from build123d import *

# Parameters (mm, degrees)
EXTRUDE_1_DEPTH         = 3
SKETCH_3_R              = 7.6
SKETCH_3_R_2            = 9.5
SKETCH_3_R_3            = 1.55
CUT_EXTRUDE_1_DEPTH     = 112.843640856
SKETCH_4_R              = 13.75
CUT_EXTRUDE_2_DEPTH     = 2
EXTRUDE_6_DEPTH         = 3
SKETCH_10_R             = 1.55
CUT_EXTRUDE_3_DEPTH     = 124.991771172
CUT_EXTRUDE_6_DEPTH     = 124.991771172
EXTRUDE_7_DEPTH         = 3
CUT_EXTRUDE_7_DEPTH     = 124.991771172
SKETCH_18_W             = 9.7
SKETCH_18_H             = 35
CUT_EXTRUDE_9_DEPTH     = 124.991771172
SKETCH_19_R             = 1.55
CUT_EXTRUDE_10_DEPTH    = 124.991771172
SKETCH_20_W             = 61.573881036
SKETCH_20_H             = 3.2
SKETCH_20_W_2           = 79.598608315
SKETCH_20_H_2           = 1.2
EXTRUDE_8_DEPTH         = 3
EXTRUDE_START           = -3
EXTRUDE_9_DEPTH         = 3
EXTRUDE_11_DEPTH        = 3
SKETCH_25_R             = 9.5
EXTRUDE_12_DEPTH        = 3
SKETCH_26_R             = 9.5
CUT_EXTRUDE_11_DEPTH    = 124.991771172
EXTRUDE_13_DEPTH        = 3
CUT_EXTRUDE_12_DEPTH    = 3
SKETCH_29_W             = 5.5
SKETCH_29_H             = 32
EXTRUDE_14_DEPTH        = 3
SKETCH_32_W             = 9.716106013
SKETCH_32_H             = 6
CUT_EXTRUDE_13_DEPTH    = 124.991771172
CUT_EXTRUDE_16_DEPTH    = 3
SKETCH_35_W             = 2.5
SKETCH_35_H             = 44.4
EXTRUDE_15_DEPTH        = 3
SKETCH_36_R             = 1.55
CUT_EXTRUDE_14691_DEPTH = 3
EXTRUDE_16_DEPTH        = 3
SKETCH_38_R             = 2.75
CUT_EXTRUDE_L_DEPTH     = 121.232106085
SKETCH_57_R             = 1.55
EXTRUDE_17_DEPTH        = 3
CUT_EXTRUDE_17_DEPTH    = 121.232106085


# Read off the part's stored shape, not the designer's step: 高级异型孔6
with BuildPart() as part:
    # 草图1 → 凸台-拉伸1 (new body)
    with BuildSketch(Plane(origin=(0, 0, 0), x_dir=(0, 0, -1), z_dir=(1, 0, 0))):
        Polygon((0, -50), (18.610302832, -39.45792997), (18.610302832, 40), (58.496702951, 40), (58.496702951, 0), (100, 0), (100, -50), align=None)
    extrude(amount=EXTRUDE_1_DEPTH)

    # 草图3 → 切除-拉伸1 (cut, through all)
    with BuildSketch(Plane.ZY):
        with Locations((-74, -24.961577338)):
            Circle(SKETCH_3_R)
        with Locations((-34.176393222, 0)):
            Circle(SKETCH_3_R_2)
        with Locations((-74, -7.461577338)):
            Circle(SKETCH_3_R_3)
        with Locations((-56.5, -24.961577338)):
            Circle(SKETCH_3_R_3)
        with Locations((-74, -42.461577338)):
            Circle(SKETCH_3_R_3)
        with Locations((-91.5, -24.961577338)):
            Circle(SKETCH_3_R_3)
    extrude(amount=-CUT_EXTRUDE_1_DEPTH, mode=Mode.SUBTRACT)

    # 草图4 → 切除-拉伸2 (cut)
    with BuildSketch(Plane.ZY):
        with Locations((-74, -24.961577338)):
            Circle(SKETCH_4_R)
    extrude(amount=-CUT_EXTRUDE_2_DEPTH, mode=Mode.SUBTRACT)

    # 草图6 → 凸台-拉伸6 (add)
    with BuildSketch(Plane.ZY):
        with BuildLine():
            Line((-102.983893987, -45.2), (-110.983893987, -45.2))
            Line((-110.983893987, -45.2), (-111, -50))
            Line((-111, -50), (-100, -50))
            Line((-100, -50), (-100, 0))
            Line((-100, 0), (-110.983893987, 0))
            Line((-110.983893987, 0), (-110.983893987, -6.8))
            Line((-110.983893987, -6.8), (-102.983893987, -6.8))
            ThreePointArc((-102.983893987, -6.8), (-101.283893987, -8.5), (-102.983893987, -10.2))
            Line((-102.983893987, -10.2), (-110.983893987, -10.2))
            Line((-110.983893987, -10.2), (-110.983893987, -41.8))
            Line((-110.983893987, -41.8), (-102.983893987, -41.8))
            ThreePointArc((-102.983893987, -41.8), (-101.283893987, -43.5), (-102.983893987, -45.2))
        make_face()
        with BuildLine():
            Line((-15.00347976, -50), (-34.686448159, -50))
            ThreePointArc((-34.686448159, -50), (-33.16855591, -50.235967767), (-31.793933119, -50.921598751))
            Line((-31.793933119, -50.921598751), (-26.580472983, -54.619128968))
            ThreePointArc((-26.580472983, -54.619128968), (-25.755699309, -55.030507559), (-24.844963959, -55.172088219))
            ThreePointArc((-24.844963959, -55.172088219), (-23.93422861, -55.030507559), (-23.109454935, -54.619128968))
            Line((-23.109454935, -54.619128968), (-17.8959948, -50.921598751))
            ThreePointArc((-17.8959948, -50.921598751), (-16.521372009, -50.235967767), (-15.00347976, -50))
        make_face()
    extrude(amount=-EXTRUDE_6_DEPTH)

    # 草图10 → 切除-拉伸3 (cut, through all)
    with BuildSketch(Plane.ZY):
        with Locations((-105.983893987, -15.2)):
            Circle(SKETCH_10_R)
        with Locations((-105.983893987, -36.8)):
            Circle(SKETCH_10_R)
    extrude(amount=-CUT_EXTRUDE_3_DEPTH, mode=Mode.SUBTRACT)

    # 草图14 → 切除-拉伸6 (cut, through all)
    with BuildSketch(Plane(origin=(3, 0, 0), x_dir=(0, 0, -1), z_dir=(1, 0, 0))):
        with BuildLine():
            Line((58.496702951, 0), (58.496702951, 40))
            Line((58.496702951, 40), (18.610302832, 40))
            Line((18.610302832, 40), (18.610302832, 18.686206016))
            ThreePointArc((18.610302832, 18.686206016), (44.493983197, 22.023278649), (58.496702951, 0))
        make_face()
    extrude(amount=-CUT_EXTRUDE_6_DEPTH, mode=Mode.SUBTRACT)

    # 草图15 → 凸台-拉伸7 (add)
    with BuildSketch(Plane(origin=(3, 0, 0), x_dir=(0, 0, -1), z_dir=(1, 0, 0))):
        with BuildLine():
            Line((18.610302832, 18.686206016), (18.610302832, -18.686206016))
            ThreePointArc((18.610302832, -18.686206016), (9.856083494, 0), (18.610302832, 18.686206016))
        make_face()
    extrude(amount=-EXTRUDE_7_DEPTH)

    # 草图16 → 切除-拉伸7 (cut, through all)
    with BuildSketch(Plane(origin=(3, 0, 0), x_dir=(0, 0, -1), z_dir=(1, 0, 0))):
        with BuildLine():
            Line((18.610302832, -18.686206016), (18.610302832, 0))
            ThreePointArc((18.610302832, 0), (34.176393222, 15.56609039), (49.742483613, 0))
            Line((49.742483613, 0), (58.496702951, 0))
            ThreePointArc((58.496702951, 0), (23.858803248, 22.023278649), (18.610302832, -18.686206016))
        make_face()
    extrude(amount=-CUT_EXTRUDE_7_DEPTH, mode=Mode.SUBTRACT)

    # 草图18 → 切除-拉伸9 (cut, through all)
    with BuildSketch(Plane.ZY):
        with Locations((-106.133893987, -26)):
            Rectangle(SKETCH_18_W, SKETCH_18_H)
    extrude(amount=-CUT_EXTRUDE_9_DEPTH, mode=Mode.SUBTRACT)

    # 草图19 → 切除-拉伸10 (cut, through all)
    with BuildSketch(Plane.ZY):
        with Locations((-105.983893987, -1.8)):
            Circle(SKETCH_19_R)
        with Locations((-105.993932098, -48.2)):
            Circle(SKETCH_19_R)
    extrude(amount=-CUT_EXTRUDE_10_DEPTH, mode=Mode.SUBTRACT)

    # 草图20 → 凸台-拉伸8 (add)
    with BuildSketch(Plane.ZY):
        with Locations((-80.196953469, 1.6)):
            Rectangle(SKETCH_20_W, SKETCH_20_H)
        with Locations((-71.200695842, -50.6)):
            Rectangle(SKETCH_20_W_2, SKETCH_20_H_2)
    extrude(amount=-EXTRUDE_8_DEPTH)

    # 草图22 → 凸台-拉伸9 (add)
    with BuildSketch(Plane.ZY.offset(EXTRUDE_START)):
        with BuildLine():
            Line((-18.610302832, 0), (-18.610302832, 25))
            Line((-18.610302832, 25), (-41.044918155, 13.968769999))
            ThreePointArc((-41.044918155, 13.968769999), (-25.948784515, 13.213993529), (-18.610302832, 0))
        make_face()
    extrude(amount=EXTRUDE_9_DEPTH)

    # 草图24 → 凸台-拉伸11 (add)
    with BuildSketch(Plane.ZY):
        Polygon((-18.610302832, 25), (-70.983893987, 3.2), (-49.410012951, 3.2), align=None)
    extrude(amount=-EXTRUDE_11_DEPTH)

    # 草图25 → 凸台-拉伸12 (add, through all)
    with BuildSketch(Plane(origin=(3, 0, 0), x_dir=(0, 0, -1), z_dir=(1, 0, 0))):
        with Locations((34.176393222, 0)):
            Circle(SKETCH_25_R)
    extrude(amount=-EXTRUDE_12_DEPTH)

    # 草图26 → 切除-拉伸11 (cut, through all)
    with BuildSketch(Plane(origin=(3, 0, 0), x_dir=(0, 0, -1), z_dir=(1, 0, 0))):
        with Locations((29.059828781, -15.2)):
            Circle(SKETCH_26_R)
    extrude(amount=-CUT_EXTRUDE_11_DEPTH, mode=Mode.SUBTRACT)

    # 草图27 → 凸台-拉伸13 (add)
    with BuildSketch(Plane.ZY):
        Polygon((-18.610302832, -10.2), (-13.610302832, -15.2), (-18.610302832, -20.2), align=None)
    extrude(amount=-EXTRUDE_13_DEPTH)

    # 草图28 → 切除-拉伸12 (cut)
    with BuildSketch(Plane.ZY):
        Polygon((-110.983893987, 3.2), (-101.283893987, 3.2), (-70.983893987, 3.2), (-95.008477086, -6.8), (-101.283893987, -6.8), (-101.283893987, -45.2), (-110.983893987, -45.2), align=None)
    extrude(amount=-CUT_EXTRUDE_12_DEPTH, mode=Mode.SUBTRACT)

    # 草图29 → 凸台-拉伸14 (add)
    with BuildSketch(Plane.ZY):
        with Locations((-104.033893987, -27.7)):
            Rectangle(SKETCH_29_W, SKETCH_29_H)
    extrude(amount=-EXTRUDE_14_DEPTH)

    # 草图32 → 切除-拉伸13 (cut, through all)
    with BuildSketch(Plane.ZY):
        with Locations((-106.141946993, -48.2)):
            Rectangle(SKETCH_32_W, SKETCH_32_H)
    extrude(amount=-CUT_EXTRUDE_13_DEPTH, mode=Mode.SUBTRACT)

    # 草图34 → 切除-拉伸16 (cut)
    with BuildSketch(Plane.ZY):
        Polygon((-103.783893987, -15.75), (-103.783893987, -12.55), (-106.783893987, -13.5), (-106.783893987, -14.8), align=None)
        Polygon((-106.783893987, -18), (-106.783893987, -19.3), (-103.783893987, -20.25), (-103.783893987, -17.05), align=None)
        Polygon((-106.783893987, -22.5), (-106.783893987, -23.8), (-103.783893987, -24.75), (-103.783893987, -21.55), align=None)
        Polygon((-106.783893987, -27), (-106.783893987, -28.3), (-103.783893987, -29.25), (-103.783893987, -26.05), align=None)
        Polygon((-106.783893987, -31.5), (-106.783893987, -32.8), (-103.783893987, -33.75), (-103.783893987, -30.55), align=None)
        Polygon((-106.783893987, -36), (-106.783893987, -37.3), (-103.783893987, -38.25), (-103.783893987, -35.05), align=None)
        Polygon((-106.783893987, -40.5), (-106.783893987, -41.8), (-103.783893987, -42.75), (-103.783893987, -39.55), align=None)
    extrude(amount=-CUT_EXTRUDE_16_DEPTH, mode=Mode.SUBTRACT)

    # 草图35 → 凸台-拉伸15 (add, through all)
    with BuildSketch(Plane.ZY):
        with Locations((-102.533893987, -29)):
            Rectangle(SKETCH_35_W, SKETCH_35_H)
    extrude(amount=-EXTRUDE_15_DEPTH)

    # 草图36 → Cut-Extrude 14691 (cut)
    with BuildSketch(Plane.ZY):
        with Locations((-93.783893987, -48.2)):
            Circle(SKETCH_36_R)
        with Locations(Location((-93.783893987, -12.9, 0), (0, 0, 180))):
            Circle(SKETCH_36_R)
        with Locations((-21.610302832, 20.501770791)):
            Circle(SKETCH_36_R)
        with Locations((-11.382694019, -47)):
            Circle(SKETCH_36_R)
    extrude(amount=-CUT_EXTRUDE_14691_DEPTH, mode=Mode.SUBTRACT)

    # 草图37 → 凸台-拉伸16 (add)
    with BuildSketch(Plane.ZY):
        Polygon((-13.610302832, -39.45792997), (-13.610302832, -42.290250896), (-18.610302832, -39.45792997), (-18.610302832, 25), (-13.610302832, 25), align=None)
    extrude(amount=-EXTRUDE_16_DEPTH)

    # 草图38 → L型支架定位孔 (cut, through all)
    with BuildSketch(Plane(origin=(3, 0, 0), x_dir=(0, 0, -1), z_dir=(1, 0, 0))):
        with Locations((93.283893987, -38.15)):
            Circle(SKETCH_38_R)
        with Locations((100.283893987, -33.15)):
            Circle(SKETCH_38_R)
    extrude(amount=-CUT_EXTRUDE_L_DEPTH, mode=Mode.SUBTRACT)

    # 高级异型孔6 outline → 高级异型孔6 (revolve, cut)
    with BuildSketch(Plane(origin=(0, -24.961577338, -56.5), x_dir=(0, 1, 0), z_dir=(0, 0, -1))):
        Polygon((1.55, 3), (1.55, 1.4), (1.7, 1.4), (3.3, 3), align=None)
    revolve(axis=Axis((0, -24.961577338, -56.5), (1, 0, 0)), mode=Mode.SUBTRACT)

    # 草图57 → 凸台-拉伸17 (add, through all)
    with BuildSketch(Plane.ZY):
        with Locations((-21.610302832, 20.501770791)):
            Circle(SKETCH_57_R)
    extrude(amount=-EXTRUDE_17_DEPTH)

    # 草图56 → 切除-拉伸17 (cut, through all)
    with BuildSketch(Plane.ZY):
        Polygon((-95.008477086, -6.8), (-18.610302832, 20.82), (-13.610302832, 20.82), (-13.610302832, 25), (-18.610302832, 25), align=None)
    extrude(amount=-CUT_EXTRUDE_17_DEPTH, mode=Mode.SUBTRACT)


solid = part.part
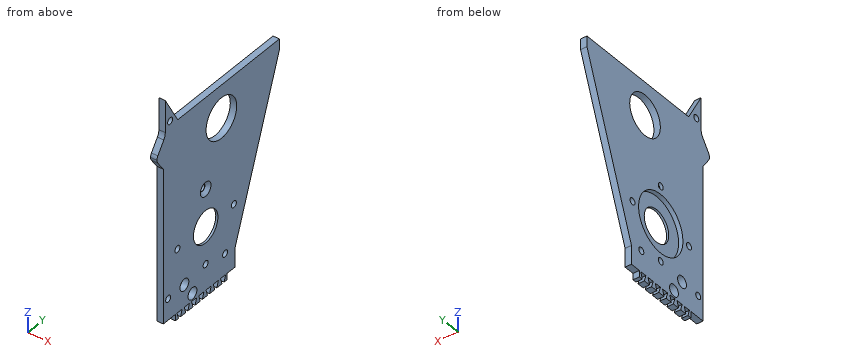
Input: part model. Units: mm. Frame: model coordinates. Coordinates: 2 decimals unless noted, no trailing zeros. Loops run counter-clockwise (first coordinate to the right, second up) from the corner with the lowest first, then second, coordinate; pieces in that order, holes last.
(1) Material intervals for probe 1 along Y at (x, z) = (1.3, -74); probe 2 along Y at (x, z) = (2.65, -74); probe 3 along Z at (x, y) = (1.2, -25.5), sorted ascending.
(2) Section C-C on y = 0. Return the cut outline in (x, z), then the cut area to 3 significant figures.
(3) Section B-B on z = -36. Return the cut outline in (x, y), then the cut area to 3 significant figures.
(4) First-contact query: pin 1 Ø0.9 at (x, z) = (1.5, -99.5) entering from +Y; pin 2 Ø0.9 at (x, z) = (1, -105) entering from -Y; pin 3 Ø3.5 at (y, z) = (-24.5, -56) entering from +X. Flat tips, straight axial feed; report the tip coordinate or a pass-through.
(5) Section A-A on z = -56.5. Return the cut outline in (x, y).
Data:
1. probe 1: y = -51.2 to -44.01, -40.91 to -38.71, -11.21 to -9.01, -5.91 to 0.8
1. probe 2: y = -51.2 to -44.01, -40.91 to -32.56, -17.36 to -9.01, -5.91 to 0.8
1. probe 3: z = -106.78 to -92.95, -90.05 to -87.74, -60.26 to -57.95, -55.05 to -13.61
2. outline: (0, -76.2) - (3, -76.2) - (3, -13.61) - (0, -13.61) - close
2. area: 188 mm2
3. outline: (0, -51.2) - (3, -51.2) - (3, -21.69) - (0, -21.69) - close; (0, -8.71) - (3, -8.71) - (3, 14.53) - (0, 14.53) - close
3. area: 158 mm2
4. pin 1: stops at y = -6.8
4. pin 2: stops at y = -43.7
4. pin 3: stops at x = 2.13
5. outline: (0, -51.2) - (3, -51.2) - (3, -28.26) - (1.4, -26.66) - (1.4, -26.51) - (0, -26.51) - close; (0, -23.41) - (1.4, -23.41) - (1.4, -23.26) - (3, -21.66) - (3, 7.12) - (0, 7.12) - close
